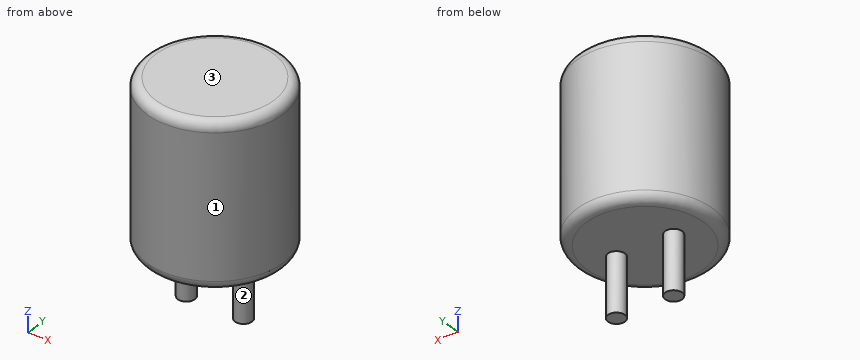
from build123d import *

# Parameters (mm, degrees)
SKETCH_R          = 3.6
PAD_DEPTH         = 8.5
FILLET_R          = 0.5
SKETCH001_R       = 0.45
PAD001_DEPTH      = 4.25
PAD001_DEPTH_BACK = 3.5


with BuildPart() as fillet_body:
    # Sketch → Pad (new body)
    with BuildSketch(Plane.XY.offset(0.1)):
        with Locations((1.5, 0)):
            Circle(SKETCH_R)
    extrude(amount=PAD_DEPTH)

    # Fillet
    fillet_edges = [fillet_body.edges().sort_by_distance(p)[0] for p in [
        (-2.1, 0, 0.1),
        (-2.1, 0, 8.6),
    ]]
    fillet(fillet_edges, radius=FILLET_R)


with BuildPart() as obj1:
    # Sketch001 → Pad001 (new body, two sides)
    with BuildSketch(Plane.XY.offset(0.5)) as pad001_sk:
        Circle(SKETCH001_R)
        with Locations((3, 0)):
            Circle(SKETCH001_R)
    extrude(amount=PAD001_DEPTH)
    extrude(pad001_sk.sketch, amount=-PAD001_DEPTH_BACK)

    # obj1: union Fillet body
    add(fillet_body.part)


solid = obj1.part
Check sheet for the modelled part. Datum: model origin and axes. Units: mm. Face numbers are marked on the shaded views. Round coordinates to 2 decimals unless told otherwise and drop trailing zeros. Loops run counter-clockwise (first coordinate to the right, second up) from the corner with the lowest first, then second, coordinate; pieces in that order, holes last. Notation, with made-up numbers: M -29.5,19 L 8.5,19 A35 ccw 8.5,58 Z; hole C 5.5,66.5 d5. An arc over 180 degrees is marked long. One line per item, written item: value.
(1) Sectioned sample at D-D, the plane z = 6. Record the cut outline in (x, y).
Computed values:
outline: C 1.5,0 d7.2
(2) Sectioned sample at A-A, the plane x = 1.5. Record the cut outline in (y, z).
Computed values:
outline: M -3.6,0.6 A0.5 ccw -3.1,0.1 L 3.1,0.1 A0.5 ccw 3.6,0.6 L 3.6,8.1 A0.5 ccw 3.1,8.6 L -3.1,8.6 A0.5 ccw -3.6,8.1 Z
(3) Sectioned sample at C-C, the plane z = -0.25. Record the cut outline in (x, y), then the cut area to 3 significant figures.
Computed values:
outline: C 0,0 d0.9; C 3,0 d0.9
area: 1.27 mm^2
(4) Thickness scan on line 1 (Z direction, x = -0.5, y = -1); line 2 (Y direction, x = 1, z = 1.75); line 3 (Y direction, x = 3.75, z = 6.5). Record the ranges inside material, lowest first.
Computed values:
line 1: z = 0.1 to 8.6
line 2: y = -3.57 to 3.57
line 3: y = -2.81 to 2.81
(5) Depth check by flat-ended pin: pin 1 Ø2 at (x, z) = (3.5, -1) entering from -Y; pin 2 Ø4 at (y, z) = (-2.5, 5) entering from +X; pin 3 Ø1.5 at (x, z) = (2.5, 1.5) entering from +Y. Enter the tip coordinate at first touch or a pass-through.
Computed values:
pin 1: stops at y = -0.45
pin 2: stops at x = 5.07
pin 3: stops at y = 3.59
(6) Release check for a two-part mould opening along X. For the marked faces 1, 2 and 3 record: +X half, -X half, draft (parallel to the pull), parting line (faces both ways), or undercut.
Computed values:
face 1: parting line
face 2: undercut
face 3: draft
(7) Sectioned sample at B-B, the plane y = 0. Record the cut outline in (x, z), then the cut area to 3 significant figures.
Computed values:
outline: M -2.1,0.6 A0.5 ccw -1.6,0.1 L -0.45,0.1 L -0.45,-3 L 0.45,-3 L 0.45,0.1 L 2.55,0.1 L 2.55,-3 L 3.45,-3 L 3.45,0.1 L 4.6,0.1 A0.5 ccw 5.1,0.6 L 5.1,8.1 A0.5 ccw 4.6,8.6 L -1.6,8.6 A0.5 ccw -2.1,8.1 Z
area: 66.6 mm^2
